Source: CAD feature listing. Evaluate the final solid. Frame: model axes, mm. Face numbers are marked on the shaded views. A direction names the side the tool comes from. Round coordinates to 2 decimals unless told otherwise and drop trailing zeros. Write each loop counter-clockwise with the first axis right and the second up, starting at its lowest first coordinate (ties: lowest second). Pieces come first, ordered by that corner, then holes. Notation, with made-up numbers: M 76,-14 L 98,-14 A27 cw 98,2 Z; hole C -15.5,66.25 d2. An arc over 180 degrees is marked long. Answer in a Markdown table with one row per item. Add a question column.
Item 1: Set-up query: the marked faces 1, 2 and 3. Return all of +Z, -Z, +X, -X, +Y, -Y with unobstructed straight access to the full face (end or side cutting, diameter ignored); none if empty.
Item 2: Cut plane B-B on x = -17.5. Give the number of separate pieces and of enclosed holes in the cut face, and give its area (3 significant figures).
Item 3: Contact query for flat-ended pins moving along their axis: pin 1 (3 mm diameter, centred on y = -20, z = -2.5, fed in from +X); pin 2 (5 mm diameter, centred on x = 35.5, z = -11.5, fed in from +Y); pin 3 (2.5 mm diameter, centred on x = -17, z = -8.5, fed in from -Y). Output: stop coordinate, or through.
Item 4: Cut plane A-A on z = -4.5. Return loops of the section in (x, y), and give its area (3 significant figures).
Item 5: Mould query, pull axis X, two halves, no side actions, for the marked faces 4, 5 and 6. Classes: released by +X, released by -X, zero draft, split by the parting line, or undercut.
Item 6: Material intervals for probe 1 along Y at (x, z) = (-18.5, -10); probe 2 along Y at (x, z) = (-15, -10.5); probe 3 along X at (y, z) = (27, -6.5) (3 decimals), sorted ascending.
from build123d import *

# Parameters (mm, degrees)
SKETCH_2_R          = 2.5
SKETCH_2_R_2        = 3
CUT_EXTRUDE_1_DEPTH = 60.99270789
CUT_EXTRUDE_2_DEPTH = 8
CHAMFER_1_SIZE      = 2


with BuildPart() as part:
    # 草图1 → 旋转1 (revolve)
    with BuildSketch(Plane(origin=(0, 0, 0), x_dir=(0, 0, -1), z_dir=(1, 0, 0))):
        Polygon((0, 41.25), (0, 22.5), (7, 22.5), (7, 8.15), (14, 8.15), (14, 41.25), align=None)
    revolve(axis=Axis((0, 0, -14), (0, 0, 1)))

    # 草图2 → 切除-拉伸1 (cut, through all)
    with BuildSketch(Plane.XY):
        with Locations((-17.5, 30.310889132)):
            Circle(SKETCH_2_R)
        with Locations((17.5, 30.310889132)):
            Circle(SKETCH_2_R)
        with Locations((35, 0)):
            Circle(SKETCH_2_R)
        with Locations((17.5, -30.310889132)):
            Circle(SKETCH_2_R)
        with Locations((-17.5, -30.310889132)):
            Circle(SKETCH_2_R)
        with Locations((-35, 0)):
            Circle(SKETCH_2_R)
        with Locations((-11.437452186, 11.437452186)):
            Circle(SKETCH_2_R_2)
        with Locations((11.437452186, 11.437452186)):
            Circle(SKETCH_2_R_2)
        with Locations((11.437452186, -11.437452186)):
            Circle(SKETCH_2_R_2)
        with Locations((-11.437452186, -11.437452186)):
            Circle(SKETCH_2_R_2)
    extrude(amount=-CUT_EXTRUDE_1_DEPTH, mode=Mode.SUBTRACT)

    # 草图3 → 切除-拉伸2 (cut)
    with BuildSketch(Plane(origin=(0, 0, -14), x_dir=(-1, 0, 0), z_dir=(0, 0, -1))):
        Polygon((-12.82346282, 30.310889132), (-15.16173141, 34.360889132), (-19.83826859, 34.360889132), (-22.17653718, 30.310889132), (-19.83826859, 26.260889132), (-15.16173141, 26.260889132), align=None)
        Polygon((19.83826859, 26.260889132), (22.17653718, 30.310889132), (19.83826859, 34.360889132), (15.16173141, 34.360889132), (12.82346282, 30.310889132), (15.16173141, 26.260889132), align=None)
        Polygon((32.66173141, -4.05), (37.33826859, -4.05), (39.67653718, 0), (37.33826859, 4.05), (32.66173141, 4.05), (30.32346282, 0), align=None)
        Polygon((19.83826859, -26.260889132), (15.16173141, -26.260889132), (12.82346282, -30.310889132), (15.16173141, -34.360889132), (19.83826859, -34.360889132), (22.17653718, -30.310889132), align=None)
        Polygon((-15.16173141, -26.260889132), (-19.83826859, -26.260889132), (-22.17653718, -30.310889132), (-19.83826859, -34.360889132), (-15.16173141, -34.360889132), (-12.82346282, -30.310889132), align=None)
        Polygon((-32.66173141, 4.05), (-37.33826859, 4.05), (-39.67653718, 0), (-37.33826859, -4.05), (-32.66173141, -4.05), (-30.32346282, 0), align=None)
    extrude(amount=-CUT_EXTRUDE_2_DEPTH, mode=Mode.SUBTRACT)

    # 倒角1
    # the kernel refuses this chamfer: 2 mm, written as the material it takes off along each edge
    with BuildSketch(Plane(origin=(0, 0, -14), x_dir=(0, 1, 0), z_dir=(1, 0, 0))) as chamfer_1_piece_1:
        Polygon((41.25, CHAMFER_1_SIZE), (41.25 - CHAMFER_1_SIZE, 0), (41.25, 0), align=None)
    revolve(axis=Axis((0, 0, -14), (0, 0, 1)), mode=Mode.SUBTRACT)
    with BuildSketch(Plane(origin=(0, 0, 0), x_dir=(0, 1, 0), z_dir=(1, 0, 0))) as chamfer_1_piece_2:
        Polygon((22.5 + CHAMFER_1_SIZE, 0), (22.5, -CHAMFER_1_SIZE), (22.5, 0), align=None)
    revolve(axis=Axis((0, 0, 0), (0, 0, 1)), mode=Mode.SUBTRACT)


solid = part.part
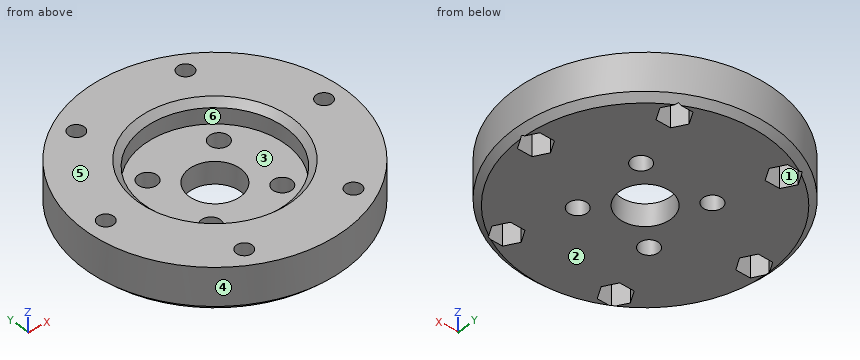
Results below:
| question | item | result |
|---|---|---|
| 1 | face 1 | -Z |
| 1 | face 2 | -Z, +X, -X, +Y, -Y |
| 1 | face 3 | +Z |
| 2 | separate pieces | 3 |
| 2 | enclosed holes | 0 |
| 2 | area | 648 mm2 |
| 3 | pin 1 | x = 36.87 |
| 3 | pin 2 | y = 24.75 |
| 3 | pin 3 | y = -38.12 |
| 4 | outline | C 0,0 d82.5; hole C -35,0 d5; hole C 0,0 d45; hole C -17.5,-30.31 d5; hole C -17.5,30.31 d5; hole C 17.5,-30.31 d5; hole C 17.5,30.31 d5; hole C 35,0 d5 |
| 4 | area | 3,640 mm2 |
| 5 | face 4 | split by the parting line |
| 5 | face 5 | zero draft |
| 5 | face 6 | undercut |
| 6 | probe 1 | -36.87 to -34.36, -26.26 to 26.26, 34.36 to 36.87 |
| 6 | probe 2 | -38.43 to -34.08, -26.54 to 26.54, 34.08 to 38.43 |
| 6 | probe 3 | -31.186 to -20.265, -14.735 to 14.735, 20.265 to 31.186 |
